Verification items for this drawing (mm, ordinates from the low corner). A direction names the side the tool comes from. Round coordinates to 2 decimals unless told otherwise and drop trailing zeros. Order: outer loops, then holes, each group sorted by start corner. A loop starts at its lowest first (then second) coordinate and runs counter-clockwise, first axis right, second up. Notation, with made-up numbers: (8, 18) -> (44, 18) arc R25 ccw to (44, 41) -> close; hole circle Ø3 at (35.25, 25). An arc over 180 degrees is marked (long way). Return JSON: item names as keys, results as strings. Group by question number.
Item 1: Sectioned sample at C-C on y = 7.5. Record the cut outline in (x, z) (1 decimal).
Item 2: Sectioned sample at A-A on x = 2.5. Record the cut outline in (y, z).
Item 3: Sectioned sample at D-D on y = 10. Record the cut outline in (x, z).
Item 4: Sectioned sample at B-B on z = 1.55. Record the cut outline in (x, y), plus the area to 3 significant figures.
Item 5: Draft check along Y on the marked faces 3, 4 and 5. Enter one of: pulls with the +Y half, pulls with the -Y half, needs draft (parallel to the pull), parting line crosses it, or undercut.
Item 6: Scan lines: probe 1 along Y at (x, z) = (8.5, 1.7) (1 decimal); probe 2 along Y at (x, z) = (12.5, 2.15); probe 3 along X at (y, z) = (7, 2.65) (1 decimal). Record each from-to range of solid material in increasing order. Write a range as from..to.
Item 7: Access from +Z, -Z, +X, -X, +Y, -Y to the whole of each face (thin tool, end or side, straight path). Record for the marked faces 1 and 2.
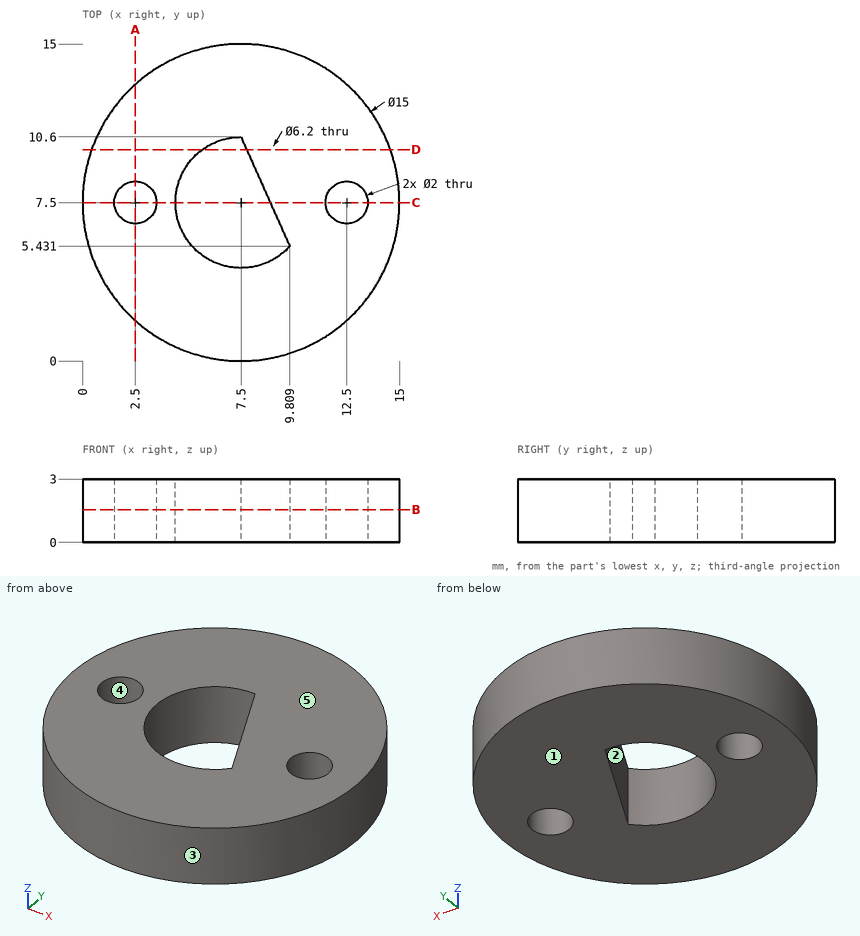
Recorded:
{
 "1": {"outline": "(0, 0) -> (1.5, 0) -> (1.5, 3) -> (0, 3) -> close; (3.5, 0) -> (4.4, 0) -> (4.4, 3) -> (3.5, 3) -> close; (8.9, 0) -> (11.5, 0) -> (11.5, 3) -> (8.9, 3) -> close; (13.5, 0) -> (15, 0) -> (15, 3) -> (13.5, 3) -> close"},
 "2": {"outline": "(1.91, 0) -> (6.5, 0) -> (6.5, 3) -> (1.91, 3) -> close; (8.5, 0) -> (13.09, 0) -> (13.09, 3) -> (8.5, 3) -> close"},
 "3": {"outline": "(0.43, 0) -> (5.67, 0) -> (5.67, 3) -> (0.43, 3) -> close; (7.77, 0) -> (14.57, 0) -> (14.57, 3) -> (7.77, 3) -> close"},
 "4": {"outline": "circle Ø15 at (7.5, 7.5); hole circle Ø2 at (2.5, 7.5); hole (7.5, 10.6) arc R3.1 ccw (long way) to (9.81, 5.43) -> close; hole circle Ø2 at (12.5, 7.5)", "area": "148 mm²"},
 "5": {"face 3": "parting line crosses it", "face 4": "undercut", "face 5": "needs draft"},
 "6": {"probe 1": "0.1..4.6, 8.4..14.9", "probe 2": "1.91..6.5, 8.5..13.09", "probe 3": "0..1.6, 3.4..4.4, 9.1..11.6, 13.4..15"},
 "7": {"face 1": "-Z, +X, -X, +Y, -Y", "face 2": "+Z, -Z"}
}
